from build123d import *

# Parameters (mm, degrees)
F0_W     = 25.4
F0_H     = 25.4
F1_DEPTH = 25.4
F2_R     = 4.940733
F3_DEPTH = 6.858
F4_R     = 2.6877
F5_DEPTH = 6.096
F6_R     = 3.488924
F7_DEPTH = 5.3848


with BuildPart() as f1:
    # F0 (on Front) → F1 (new body)
    with BuildSketch(Plane.XZ):
        with Locations((0.491789, -0.80908)):
            Rectangle(F0_W, F0_H)
    extrude(amount=F1_DEPTH)

    # F2 (on face) → F3 (join)
    with BuildSketch(Plane.XY.offset(11.89092)):
        with Locations((0, -10.92047)):
            Circle(F2_R)
    extrude(amount=F3_DEPTH)

    # F4 (on face) → F5 (join)
    with BuildSketch(Plane.XY.offset(11.89092)):
        with Locations((-3.695844, -20.576853)):
            Circle(F4_R)
    extrude(amount=F5_DEPTH)

    # F6 (on face) → F7 (join)
    with BuildSketch(Plane.XY.offset(11.89092)):
        with Locations((6.692471, -19.577978)):
            Circle(F6_R)
    extrude(amount=F7_DEPTH)


solid = f1.part
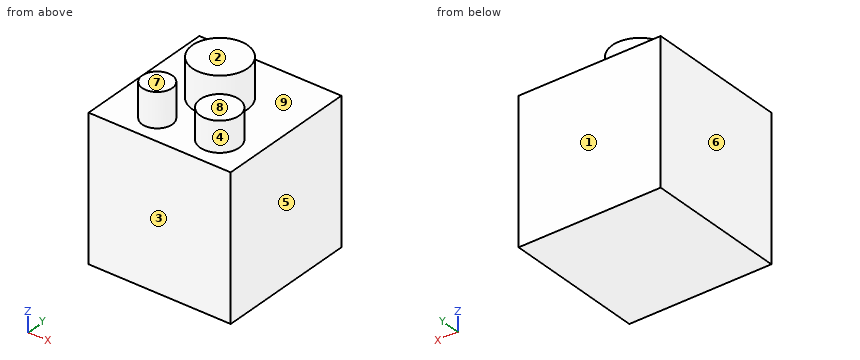
Work out the finished part from the listing and answer in its coordinate system (mm). Face numbers are marked on the shaded views. A direction names the side the tool comes from. Give positions to 0.01 mm unless a question says otherwise; leave off trailing zeros. Write each loop counter-clockwise with the first axis right and the second up, starting at its lowest first coordinate (ties: lowest second). Pieces come first, ordered by that corner, then holes. Notation, with made-up numbers: (5.5, 56.5) - (31.5, 56.5) arc R29 ccw to (31.5, 91.5) - close; hole circle Ø6 at (58.5, 48). An arc over 180 degrees is marked (long way). One line per item, written item: value. Start each with the question number.
1. Find section D-D (x = -8). Write down the section's boundary in (y, z).
2. For a pull along Y with two mould halves and no side action, classify the marked faces 1, 2, 3 and 4 as +Y half, -Y half, draft (parallel to the pull), parting line (faces both ways), or undercut.
3. Given pin 1 (7.5 mm diameter, centred on x = 8, y = -18, fed in from +Z); pin 2 (2 mm diameter, centred on y = -13, z = 14.5, fed in from +X); pin 3 (6 mm diameter, centred on x = -4, y = -19.5, fed in from +Z), each flat-ended and moving along its own axis, determine where each tip first touches the part or whether it passes through.
4. Find section A-A (x = 0). Write down the section's boundary in (y, z).
5. Find section C-C (z = 15). Write down the section's boundary in (x, y).
6. For the marked faces 5, 6, 7, 8 and 9, determine the directions among +Z, -Z, +X, -X, +Y, -Y from which every point of the face is accessible in a straight line to the end or side of a thin tool.
7. Consider probe 1 along Z at (x, y) = (-8.5, -22); probe 2 along Z at (x, y) = (7.5, -20.75). Determine where each line is inside the solid, lowest interval first.
8. Find section B-B (y = -13.75). Write down the section's boundary in (x, z), then the cut area to 3 significant figures.
Geometry results:
1. outline: (-25.4, -13.51) - (0, -13.51) - (0, 11.89) - (-25.4, 11.89) - close
2. face 1: +Y half
2. face 2: draft
2. face 3: -Y half
2. face 4: undercut
3. pin 1: z = 17.28
3. pin 2: x = 4.82
3. pin 3: z = 17.99
4. outline: (-25.4, -13.51) - (0, -13.51) - (0, 11.89) - (-5.98, 11.89) - (-5.98, 18.75) - (-15.86, 18.75) - (-15.86, 11.89) - (-25.4, 11.89) - close
5. outline: circle Ø5.38 at (-3.7, -20.58); circle Ø9.88 at (0, -10.92); circle Ø6.98 at (6.69, -19.58)
6. face 5: +Z, -Z, +X, +Y, -Y
6. face 6: +Z, -Z, -X, +Y, -Y
6. face 7: +Z, +X, -X, -Y
6. face 8: +Z, +X, -Y
6. face 9: +Z
7. probe 1: -13.51 to 11.89
7. probe 2: -13.51 to 17.28
8. outline: (-12.21, -13.51) - (13.19, -13.51) - (13.19, 11.89) - (4.05, 11.89) - (4.05, 18.75) - (-4.05, 18.75) - (-4.05, 11.89) - (-12.21, 11.89) - close
8. area: 701 mm2
